Geometry check sheet. Reference: the model listing, model coordinates, mm. Face numbers are marked on the shaded views. A direction names the side the tool comes from. Round coordinates to 2 decimals unless told otherwise and drop trailing zeros. Write each loop counter-clockwise with the first axis right and the second up, starting at its lowest first coordinate (ties: lowest second). Pieces come first, ordered by that corner, then holes. Notation, with made-up numbers: (-36.75, 42) - (20.25, 42) arc R15 cw to (20.25, 67) - close; hole circle Ø5 at (70, -39). An arc over 180 degrees is marked (long way). Return JSON: item names as keys, results as strings.
```python
from build123d import *

# Parameters (mm, degrees)
SKETCH1_R           = 4
BOSS_EXTRUDE3_DEPTH = 30
SKETCH3_W           = 30
SKETCH3_H           = 30
BOSS_EXTRUDE4_DEPTH = 10
SKETCH4_R           = 3
CUT_EXTRUDE1_DEPTH  = 10
BOSS_EXTRUDE5_START = -5
SKETCH5_R           = 4
BOSS_EXTRUDE5_DEPTH = 5
FILLET2_R           = 1


with BuildPart() as part:
    # Sketch1 → Boss-Extrude3 (new body)
    with BuildSketch(Plane(origin=(0, 0, 0), x_dir=(0, 0, -1), z_dir=(1, 0, 0))):
        with BuildLine():
            Line((-7, 0), (-7, -20))
            Line((-7, -20), (7, -20))
            Line((7, -20), (7, 0))
            ThreePointArc((7, 0), (0, 7), (-7, 0))
        make_face()
        Circle(SKETCH1_R, mode=Mode.SUBTRACT)
    extrude(amount=BOSS_EXTRUDE3_DEPTH)

    # Sketch3 → Boss-Extrude4 (add)
    with BuildSketch(Plane.XZ.offset(20)):
        with Locations((15, 0)):
            Rectangle(SKETCH3_W, SKETCH3_H)
    extrude(amount=BOSS_EXTRUDE4_DEPTH)

    # Sketch4 → Cut-Extrude1 (cut)
    with BuildSketch(Plane(origin=(0, -20, 0), x_dir=(1, 0, 0), z_dir=(0, 1, 0))):
        with Locations(Location((15, 11, 0), (0, 0, 270))):
            Circle(SKETCH4_R)
        with Locations(Location((15, -11, 0), (0, 0, 270))):
            Circle(SKETCH4_R)
    extrude(amount=-CUT_EXTRUDE1_DEPTH, mode=Mode.SUBTRACT)

    # Sketch5 → Boss-Extrude5 (add)
    with BuildSketch(Plane(origin=(30, 0, 0), x_dir=(0, 0, -1), z_dir=(1, 0, 0)).offset(BOSS_EXTRUDE5_START)):
        Circle(SKETCH5_R)
    extrude(amount=BOSS_EXTRUDE5_DEPTH)

    # Fillet2
    fillet2_edges = [part.edges().sort_by_distance(p)[0] for p in [
        (30, -10, -7),
        (30, -20, -11),
        (30, -20, 11),
        (30, -25, -15),
        (15, -20, 15),
        (30, -25, 15),
        (15, -20, -15),
        (30, -30, 0),
        (30, 7, 0),
        (30, -10, 7),
    ]]
    fillet(fillet2_edges, radius=FILLET2_R - 0.0001)  # a hair under: the kernel refuses the full size


solid = part.part
```
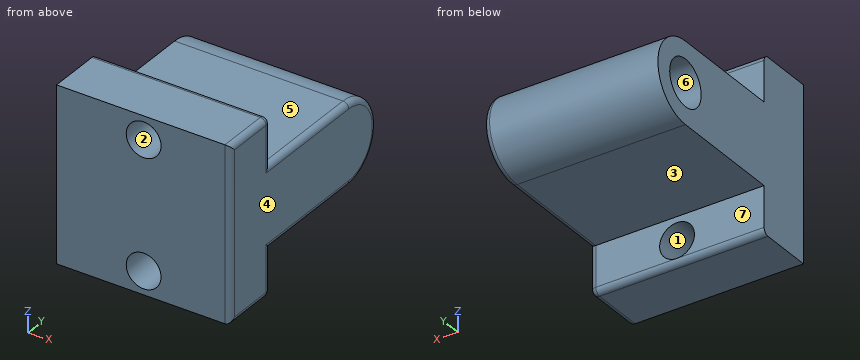
(1) Release check for a two-part mould opening along X. For the marked faces 1, 2, 3 and 4 record: pulls with the +X half, pulls with the -X half, needs draft (parallel to the pull), parting line crosses it, or undercut.
Response values:
{"face 1": "undercut", "face 2": "undercut", "face 3": "needs draft", "face 4": "pulls with the +X half"}
(2) Access from +Z, -Z, +X, -X, +Y, -Y to the whole of each face (thin tool, end or side, straight path). Record for the marked faces 5, 6 and 7.
Response values:
{"face 5": "+Z, +X, -X, +Y", "face 6": "-X", "face 7": "-Z, +X, -X, +Y"}
(3) Gauge pin test, flat ends, axial feed: pin 1 (6 mm diameter, centred on x = 18, y = -8.5, fed in from -Z); pin 2 (12 mm diameter, centred on x = 16, z = -10.5, fed in from +Y); pin 3 (10 mm diameter, centred on x = 19.5, y = -9, fed in from +Z). Record the tip position at first contact, or that the pin passes through.
Response values:
{"pin 1": "stops at z = -7", "pin 2": "stops at y = 5.36", "pin 3": "stops at z = 7"}
(4) Material ranges on line 1 along X through (y, z) = (-22.75, -11); line 2 along Y through (x, z) = (12, -12.75); line 3 along Z through (x, y) = (4, -17), recorded low to high. Write a range as [from, to].
Response values:
{"line 1": "x = [0, 12], [18, 30]", "line 2": "y = [-30, -20]", "line 3": "z = [-7, 7]"}
(5) Section check A-A, the plane x = 15. Give the number of separate pieces and of enclosed holes in the cut face, plus the area to 3 significant figures.
Response values:
{"separate pieces": "3", "enclosed holes": "1", "area": "486 mm^2"}
(6) Section check C-C, the plane z = 11. Enter the section's corners in (x, y), plus the area to 3 significant figures.
Response values:
{"outline": "(0, -30) - (12, -30) - (12, -20) - (0, -20) - close; (18, -30) - (29, -30) arc R1 ccw to (30, -29) - (30, -21) arc R1 ccw to (29, -20) - (18, -20) - close", "area": "240 mm^2"}
(7) Section check D-D, the plane z = 0. Enter the section's corners in (x, y), plus the area to 3 significant figures.
Response values:
{"outline": "(0, -30) - (29, -30) arc R1 ccw to (30, -29) - (30, 6) arc R1 ccw to (29, 7) - (0, 7) - (0, 4) - (25, 4) - (25, -4) - (0, -4) - close", "area": "910 mm^2"}
(8) Section check B-B, the plane y = -23. Enter the section's corners in (x, z), plus the area to 3 significant figures.
Response values:
{"outline": "(0, -15) - (29, -15) arc R1 ccw to (30, -14) - (30, 14) arc R1 ccw to (29, 15) - (0, 15) - close; hole circle Ø6 at (15, -11); hole circle Ø6 at (15, 11)", "area": "843 mm^2"}
